Work out the finished part from the listing and answer in its coordinate system (mm). Face numbers are marked on the shaded views. A direction names the side the tool comes from. Coordinates: 2 decimals unless noted, no trailing zeros. Order: outer loops, then holes, each group sorted by start corner. A loop starts at its lowest first (then second) coordinate and runs counter-clockwise, first axis right, second up.
1. A tool of negligible diameter and unlimited length cuts with its end or side. For the marked faces 1 and 2, from which of +Z, -Z, +X, -X, +Y, -Y can it reach the whole face along a straight path? Write none if from no direction.
2. Flat-ended cylindrical pins translate along their axes: pin 1 Ø6 at (x, y) = (-4, 1.5) entering from +Z; pin 2 Ø2 at (x, y) = (-3, 5.5) entering from -Z. Find the tip coordinate at first contact, or state that the pin passes through.
3. The part is cut by section B-B, the plane x = 2.5. Give the vertices of the cut face in (y, z) (3 decimals).
4. Determine the mould class of the marked faces 3, 4 and 5 for opening direction Y: +Y half, -Y half, draft (parallel to the pull), parting line (faces both ways), or undercut.
5. The part is cut by section C-C, the plane y = -20.5. Give the vertices of the cut face in (x, z).
6. The part is cut by section A-A, the plane z = 5.5. Give the vertices of the cut face in (x, y), then the cut area to 3 significant figures.
7. Find the intervals of material crossed by probe 1 along X at (y, z) = (-3, 2); probe 2 along X at (y, z) = (-0.5, 2.5); probe 3 along Z at (x, y) = (-8, -3), in increasing order.
8. The part is cut by section D-D, the plane z = 8. Give the vertices of the cut face in (x, y).
```python
from build123d import *

# Parameters (mm, degrees)
F1_DEPTH    = 12.7
F2_T1_DEPTH = 115.269941864
F2_T3_DEPTH = 104.1696304448
F2_T5_DEPTH = 104.1696304448
F2_T7_DEPTH = 115.269941864
F3_T        = -1.905


# Not quite as in the source:
# - a fillet or chamfer that OpenCascade refuses, or shapes differently, is made with other operations: its cross-section is extruded or revolved along the edge and cut away or added


with BuildPart() as f1:
    # F0 (on Top) → F1 (new body)
    with BuildSketch(Plane.XY):
        Polygon((16.3001076085, 0), (0, 25.4906731501), (-16.3001076085, 0), (0, -38.0093268499), align=None)
    extrude(amount=F1_DEPTH)

    # F2: chamfer of 14.351 x 12.9216984397 on 4 edges, made by hand

    # F2_s2 → F2_t1 (cut)
    with BuildSketch(Plane(origin=(-28.3337655113, -66.0699536514, 0), x_dir=(0, 0, 1), z_dir=(0.3941316562, 0.9190539906, 0))):
        Polygon((-0.2216984397, 14.980678944), (12.7, 0.629678944), (12.7, 14.980678944), align=None)
    extrude(amount=F2_T1_DEPTH, mode=Mode.SUBTRACT)

    # F2_s4 → F2_t3 (cut)
    with BuildSketch(Plane(origin=(24.6401842719, -38.5331740573, 0), x_dir=(0, 0, 1), z_dir=(-0.5387272021, 0.8424802679, 0))):
        Polygon((-0.2216984397, 13.7325190245), (12.7, -0.6184809755), (12.7, 13.7325190245), align=None)
    extrude(amount=F2_T3_DEPTH, mode=Mode.SUBTRACT)

    # F2_s6 → F2_t5 (cut)
    with BuildSketch(Plane(origin=(31.4788292763, 49.227684105, 0), x_dir=(0, 0, 1), z_dir=(-0.5387272021, -0.8424802679, 0))):
        Polygon((-0.2216984397, 13.7325190245), (12.7, -0.6184809755), (12.7, 13.7325190245), align=None)
    extrude(amount=F2_T5_DEPTH, mode=Mode.SUBTRACT)

    # F2_s8 → F2_t7 (cut)
    with BuildSketch(Plane(origin=(-17.0977675905, 39.8693464092, 0), x_dir=(0, 0, 1), z_dir=(0.3941316562, -0.9190539906, 0))):
        Polygon((-0.2216984397, 14.980678944), (12.7, 0.629678944), (12.7, 14.980678944), align=None)
    extrude(amount=F2_T7_DEPTH, mode=Mode.SUBTRACT)

    # F3
    f3_openings = [f1.faces().sort_by_distance(p)[0] for p in [
        (0, -4.124591, 0),
    ]]
    offset(amount=F3_T, openings=f3_openings)


solid = f1.part
```
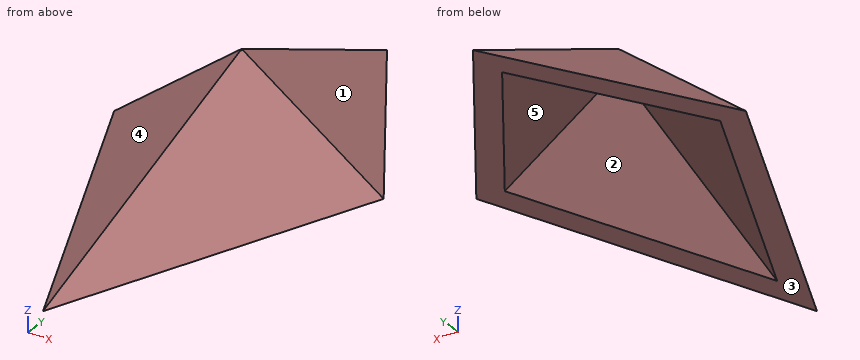
Geometry says:
1. face 1: +Z, +X, +Y
1. face 2: -Z
2. pin 1: stops at z = 11.08
2. pin 2: stops at z = 3.74
3. outline: (-31.555, 0) - (-24.332, 0) - (-1.133, 8.233) - (15.839, 0) - (21.124, 0) - (-1.133, 10.796) - close
4. face 3: draft
4. face 4: -Y half
4. face 5: undercut
5. outline: (-7.24, 0) - (-4.14, 0) - (0, 3.43) - (4.14, 0) - (7.24, 0) - (0, 5.99) - close
6. outline: (-9.13, -0.59) - (0, -21.89) - (9.13, -0.59) - (0, 13.7) - close; hole (-5.92, -0.85) - (0, -14.66) - (5.92, -0.85) - (0, 8.41) - close
6. area: 188 mm2
7. probe 1: x = -12.33 to -9.23, 9.23 to 12.33
7. probe 2: x = -12.8 to -9.65, 9.65 to 12.8
7. probe 3: z = 3.02 to 5.58
8. outline: (-6, -0.85) - (0, -14.84) - (6, -0.85) - (0, 8.54) - close; hole (-2.79, -1.11) - (0, -7.62) - (2.79, -1.11) - (0, 3.26) - close
